Autodesk Inventor part; units mm, degrees
ref_plane "YZ Plane" through (0, 0, 0) normal (1, 0, 0) x (0, 1, 0)
ref_plane "XZ Plane" through (0, 0, 0) normal (0, 1, 0) x (-1, 0, 0)
ref_plane "XY Plane" through (0, 0, 0) normal (0, 0, 1) x (1, 0, 0)
sketch "スケッチ1" plane through (0, 0, 0) normal (0, 0, 1) x (1, 0, 0)
  circle A0 centre (0, 0) radius 29
  line L0 (-9.25, 29) -> (9.25, 29)
  line L1 (9.25, 29) -> (9.25, 0)
  line L2 (9.25, 0) -> (-9.25, 0)
  line L3 (-9.25, 0) -> (-9.25, 29)
  line L4 (-9.25, 22.5) -> (9.25, 22.5)
  arc A1 (-9.25, 17.5148) -> (9.25, 17.5148) centre (0, 45) ccw
  arc A2 (-9.25, 15.9365) -> (9.25, 15.9365) centre (0, 45) ccw
  point P0 (9.25, 27.4852)
  point P1 (-9.25, 27.4852)
  point P2 (0, 22.5)
  point P3 (0, 22.5)
  dimension "d0" = 58
  dimension "d1" = 18.5
  dimension "d2" = 6.5
  dimension "d9" = 1.5
extrude "押し出し3" add sketch "スケッチ1" along normal blind 6.5 contours A0 L3 L2 L1 | L1 L4 L3 A0 | L1 A1 L3 L4 | L1 A2 L3 A1 | L1 L2 L3 A2
extrude "押し出し4" cut sketch "スケッチ1" along normal blind 6.5 contours L1 L4 L3 A0 | L1 A1 L3 L4 | L1 A2 L3 A1
pattern_circular "円形状パターン1" count 5 over 360 about axis through (0, 0, -10) along (0, 0, 1) of "押し出し4"
sketch "スケッチ4" plane through (0, 0, 0) normal (0, 0, -1) x (-1, 0, 0)
  arc A0 (-9.25, 27.4852) -> (-23.2816, 17.2907) centre (0, 0) ccw
  circle A1 centre (0, 0) radius 29
  line L0 (-9.25, 15.9365) -> (-9.25, 27.4852) construction
  arc A2 (-9.25, 15.9365) -> (9.25, 15.9365) centre (0, 45) ccw construction
  line L1 (9.25, 27.4852) -> (9.25, 15.9365) construction
  line L2 (40.6, 0) -> (-40.6, 0) construction
  line L3 (-9.25, -15.9365) -> (-9.25, -27.4852)
  arc A3 (9.25, -15.9365) -> (-9.25, -15.9365) centre (0, -45) ccw
  line L4 (9.25, -27.4852) -> (9.25, -15.9365)
  point P0 (-9.25, 27.4852)
  point P1 (-23.2816, 17.2907)
extrude "押し出し5" add sketch "スケッチ4" along normal blind 6.5
extrude "押し出し6" cut sketch "スケッチ4" along normal blind 6.5 contours L3 A3 L4 A1
pattern_circular "円形状パターン2" count 5 over 360 about axis through (0, 0, -10) along (0, 0, 1) of "押し出し6"
properties part number "base" material "ゴム"
Source: CAD feature listing. Evaluate the final solid. Frame: model axes, mm. A direction names the side the tool comes from. Give positions to 0.01 mm unless a question says otherwise; leave off trailing zeros. Order: outer loops, then holes, each group sorted by start corner. A loop starts at its lowest first (then second) coordinate and runs counter-clockwise, first axis right, second up.
(1) Pull-direction query (X, two-part tool) for faces 4 (the face through (8.417, 11.808, -3.204)), 5 (the face through (0, 0, 6.5)), 6 (the face through (-23.43, -2.113, 3.204)), 7 (the face through (27.62, -8.84, 3.2)); classes: +X half, -X half, draft (parallel to the pull), parting line (faces both ways), or undercut.
(2) Access query for faces 1 (the face through (-23, 7, 0)), 2 (the face through (-13.75, 4.61, 3.2)), 3 (the face through (23, 7, 0)). Directions: +Z, -Z, +X, -X, +Y, -Y. A direction counts if a zero-diameter tool reaches every point of the face in a straight line with its end or side. Return the directions, or none.
(3) Section query D-D (z = -3). Return the cut outline in (x, y).
(4) Contact query for flat-ended pins moving along their axis: P1, Ø2, axis at y = -20.5, z = -5, coming from the +X side; P2, Ø1.5, axis at y = -20, z = -5, coming from the +X side; P3, Ø14.5, axis at x = -14.5, y = -17, coming from the +Z side; P4, Ø1.5, axis at x = 15, y = 12.5, coming from the -Z side (1 decimal). Output: stop coordinate, or through.
(5) Section query B-B (x = 3). Return the cut outline in (y, z), plus the area to 3 significant figures.
(6) Material intervals for line 1 along Y through (x, z) = (0, 5.5); line 2 along Z through (x, y) = (-23, -12); line 3 along X through (y, z) = (10, -5), sorted ascending.
(7) Section query C-C (x = -19.5). Return the cut outline in (y, z), plus the area to 3 significant figures.
(8) Section query A-A (y = -3). Return the cut outline in (x, z).
Outcome:
1. face 4: undercut
1. face 5: draft
1. face 6: undercut
1. face 7: +X half
2. face 1: +Z, -X
2. face 2: +Z
2. face 3: +Z, +X
3. outline: (-29, 0.3) - (-18.01, 3.87) arc R30.5 cw to (-12.3, -13.72) - (-23.28, -17.29) arc R29 ccw to (-9.25, -27.49) - (-9.25, -15.94) arc R30.5 cw to (9.25, -15.94) - (9.25, -27.49) arc R29 ccw to (23.28, -17.29) - (12.3, -13.72) arc R30.5 cw to (18.01, 3.87) - (29, 0.3) arc R29 ccw to (23.64, 16.8) - (16.85, 7.46) arc R30.5 cw to (1.88, 18.33) - (8.67, 27.67) arc R29 ccw to (-8.67, 27.67) - (-1.88, 18.33) arc R30.5 cw to (-16.85, 7.46) - (-23.64, 16.8) arc R29 ccw to start
4. P1: stops at x = 21.47
4. P2: stops at x = 21.69
4. P3: stops at z = 0
4. P4: passes through
5. outline: (-28.84, 0) - (-19.87, 0) - (-19.87, 6.5) - (-28.84, 6.5) - close; (-16.9, 0) - (-14.65, 0) - (-14.65, -6.5) - (16.9, -6.5) - (16.9, 0) - (14.65, 0) - (14.65, 6.5) - (-16.9, 6.5) - close; (19.87, -6.5) - (28.84, -6.5) - (28.84, 0) - (19.87, 0) - close
5. area: 527 mm2
6. line 1: y = -29 to 14.5
6. line 2: z = 0 to 6.5
6. line 3: x = -27.22 to -18.7, -11.19 to 11.19, 18.7 to 27.22
7. outline: (-21.47, -6.5) - (-16.06, -6.5) - (-16.06, 0) - (-21.47, 0) - close; (-11.1, 0) - (-3.39, 0) - (-3.39, 6.5) - (-11.1, 6.5) - close; (3.39, -6.5) - (11.1, -6.5) - (11.1, 0) - (3.39, 0) - close; (16.06, 0) - (21.47, 0) - (21.47, 6.5) - (16.06, 6.5) - close
7. area: 171 mm2
8. outline: (-28.84, 0) - (-20.7, 0) - (-20.7, 6.5) - (-28.84, 6.5) - close; (-17.41, 0) - (-14.31, 0) - (-14.31, -6.5) - (14.31, -6.5) - (14.31, 0) - (17.41, 0) - (17.41, 6.5) - (-17.41, 6.5) - close; (20.7, 0) - (28.84, 0) - (28.84, 6.5) - (20.7, 6.5) - close
